Part model, mm, in its own coordinate system. A direction names the side the tool comes from. Give positions to 0.01 mm unless a question says otherwise; leave off trailing zeros. Order: outer loops, then holes, each group sorted by start corner. A loop starts at its lowest first (then second) coordinate and runs counter-clockwise, first axis right, second up. Notation, with made-up numbers: M -30,50 L -11,50 A27 ccw -11,79 Z; hole C 34,-2 d9. An arc over 180 degrees is marked long. Return JSON: item names as keys, results as strings.
from build123d import *

# Parameters (mm, degrees)
BOSS_EXTRUDE1_DEPTH = 9.525
CUT_EXTRUDE1_DEPTH  = 71.061798614
FILLET1_R           = 1.5875


with BuildPart() as part:
    # Sketch1 → Boss-Extrude1 (new body)
    with BuildSketch(Plane(origin=(0, 0, 0), x_dir=(1, 0, 0), z_dir=(0, 1, 0))):
        Polygon((0, 0), (0, 50.8), (3.5, 50.8), (3.5, 3.5), (47.3, 3.5), (47.3, 0), align=None)
    extrude(amount=BOSS_EXTRUDE1_DEPTH)

    # Sketch2 → Cut-Extrude1 (cut, through all)
    with BuildSketch(Plane(origin=(0, 9.525, 0), x_dir=(1, 0, 0), z_dir=(0, 1, 0))):
        Polygon((3.5, 41.3), (1.9125, 41.3), (1.9125, 3.5), (1.9125, 1.9125), (41.3, 1.9125), (41.3, 3.5), (3.5, 3.5), align=None)
    extrude(amount=-CUT_EXTRUDE1_DEPTH, mode=Mode.SUBTRACT)

    # Fillet1
    fillet1_edges = [part.edges().sort_by_distance(p)[0] for p in [
        (41.3, 4.7625, -1.9125),
        (1.9125, 4.7625, -1.9125),
        (1.9125, 4.7625, -41.3),
    ]]
    fillet(fillet1_edges, radius=FILLET1_R - 0.0001)  # a hair under: the kernel refuses the full size


solid = part.part
Q1. Pin check, flat tips, straight feed: pin 1 (4 mm diameter, centred on x = 8, y = 4.5, fed in from -Z); pin 2 (5 mm diameter, centred on x = 44.5, y = 6.5, fed in from -Z). Stop position of each tip, or through.
Established:
{"pin 1": "stops at z = -1.91", "pin 2": "stops at z = -3.5"}
Q2. Two-plate mould, pull along X, no slides. Class faces 4 (the cylindrical face through (40.85, 4.7, -2.39)), 5 (the flat face through (1.912, 5, -22)), 6 (the flat face through (2, 5, -50.8)): +X half, -X half, draft (parallel to the pull), parting line (faces both ways), or undercut.
Established:
{"face 4": "undercut", "face 5": "+X half", "face 6": "draft"}
Q3. Probe line 1 along X through (y, z) = (6.5, -38); line 2 along Z through (x, y) = (23, 2); line 3 along X through (y, z) = (1.25, -42.5). List the from-to ranges inside material, lowest first.
Established:
{"line 1": "x = 0 to 1.91", "line 2": "z = -1.91 to 0", "line 3": "x = 0 to 3.5"}
Q4. 3-axis set-ups, long thin cutter, end or side, ignore diameter. For faces 1 (the flat face through (21, 5, -1.912)), 2 (the flat face through (44, 5, -3.5)), 3 (the cylindrical face through (2.365, 4.696, -40.823)): which of +Z, -Z, +X, -X, +Y, -Y reach the whole face in a straight line?
Established:
{"face 1": "-Z, +Y, -Y", "face 2": "-Z, +X, +Y, -Y", "face 3": "+X, +Y, -Y"}
Q5. Band-saw the part on C-C (z = -14). Give the cut face in (x, y) (1 decimal).
Established:
{"outline": "M 0,0 L 1.9,0 L 1.9,9.5 L 0,9.5 Z"}
Q6. Band-saw the part on B-B (x = 19.5). Give the cut face in (y, z) (1 decimal), then the cut area to 3 significant figures.
Established:
{"outline": "M 0,-1.9 L 9.5,-1.9 L 9.5,0 L 0,0 Z", "area": "18.2 mm²"}
